Input: part model. Units: mm. Frame: model coordinates. A direction names the side the tool comes from. Coordinates: 2 decimals unless noted, no trailing zeros. Order: outer loops, then holes, each group sorted by start corner. A loop starts at its lowest first (then second) coordinate and runs counter-clockwise, first axis right, second up. Notation, with made-up numbers: (63, 83.5) -> (70, 83.5) arc R26 ccw to (70, 120.5) -> close; hole circle Ø4 at (79, 22.5). An arc over 180 degrees is marked (long way). Use one line per item in the form item = value. Start each with the question number.
1) Section query D-D on z = -7.5. Output: boundary loops of the cut face in (x, y), then the cut area to 3 significant figures.
2) Pin query (flat end, axial travel): pin 1 (5.5 mm diameter, centred on y = 9, z = -8, fed in from +X); pin 2 (7.5 mm diameter, centred on x = 5.5, y = 9.5, fed in from -Z); pin 3 (5 mm diameter, centred on x = -4, y = 8, fed in from -Z). Return the tip coordinate at first contact, or that it passes through.
3) Section query A-A on y = 14.25. Output: boundary loops of the cut face in (x, z), then the cut area to 3 significant figures.
4) Section query B-B on x = -21.5. Output: boundary loops of the cut face in (y, z), then the cut area to 3 significant figures.
5) Section query C-C on y = 3. Output: boundary loops of the cut face in (x, z).
6) Ray query, line 1 along X through (y, z) = (2.55, -18); line 2 along Y through (x, z) = (4, 4.5); line 3 along X through (y, z) = (12.5, 9). Return the intervals inside material, ascending.
7) Access query for faces 1 (the flat face through (-17, 10, 14)), 2 (the flat face through (-15, 10, 18.5)), 3 (the flat face through (15, 10, 16)), 4 (the flat face through (10, 10, 13.5)), 5 (the flat face through (17, 10, -1.5)). Directions: +Z, -Z, +X, -X, +Y, -Y. A direction counts if a zero-diameter tool reaches every point of the face in a straight line with its end or side. Return the directions, or none.
from build123d import *

# Parameters (mm, degrees)
ESQUISSE1_W        = 50
ESQUISSE1_H        = 43
ESQUISSE1_R        = 2
BOSS_EXTRU_1_DEPTH = 5
ESQUISSE2_W        = 5
ESQUISSE2_H        = 10
ESQUISSE2_H_2      = 7
ESQUISSE2_W_2      = 7
ESQUISSE2_H_3      = 5
ESQUISSE2_H_4      = 11
ESQUISSE2_W_3      = 10
BOSS_EXTRU_2_DEPTH = 15


with BuildPart() as part:
    # Esquisse1 → Boss.-Extru.1 (new body)
    with BuildSketch(Plane(origin=(0, 0, 0), x_dir=(1, 0, 0), z_dir=(0, 1, 0))):
        Rectangle(ESQUISSE1_W, ESQUISSE1_H)
        with Locations(Location((-21.5, 18, 0), (0, 0, 270))):
            Circle(ESQUISSE1_R, mode=Mode.SUBTRACT)
        with Locations(Location((21.5, 18, 0), (0, 0, 90))):
            Circle(ESQUISSE1_R, mode=Mode.SUBTRACT)
        with Locations(Location((21.5, -18, 0), (0, 0, 270))):
            Circle(ESQUISSE1_R, mode=Mode.SUBTRACT)
        with Locations(Location((-21.5, -18, 0), (0, 0, 90))):
            Circle(ESQUISSE1_R, mode=Mode.SUBTRACT)
    extrude(amount=BOSS_EXTRU_1_DEPTH)

    # Esquisse2 → Boss.-Extru.2 (add)
    with BuildSketch(Plane(origin=(0, 0, 0), x_dir=(1, 0, 0), z_dir=(0, 1, 0))):
        with Locations((-14.5, -13.5)):
            Rectangle(ESQUISSE2_W, ESQUISSE2_H)
        with Locations((-14.5, 8)):
            Rectangle(ESQUISSE2_W, ESQUISSE2_H_2)
        with Locations((4.5, 16)):
            Rectangle(ESQUISSE2_W_2, ESQUISSE2_H_3)
        with Locations((17.5, -4)):
            Rectangle(ESQUISSE2_W_2, ESQUISSE2_H_4)
        with Locations((10, -16)):
            Rectangle(ESQUISSE2_W_3, ESQUISSE2_H_3)
        with Locations((-3, -16)):
            Rectangle(ESQUISSE2_W_3, ESQUISSE2_H_3)
    extrude(amount=BOSS_EXTRU_2_DEPTH)


solid = part.part
Answers below:
q1.outline = (-25, 0) -> (25, 0) -> (25, 5) -> (-12, 5) -> (-12, 15) -> (-17, 15) -> (-17, 5) -> (-25, 5) -> close
q1.area = 300 mm^2
q2.pin_1 = -12
q2.pin_2 = -18.5
q2.pin_3 = 13.5
q3.outline = (-17, -11.5) -> (-12, -11.5) -> (-12, -4.5) -> (-17, -4.5) -> close; (-17, 8.5) -> (-12, 8.5) -> (-12, 18.5) -> (-17, 18.5) -> close; (-8, 13.5) -> (2, 13.5) -> (2, 18.5) -> (-8, 18.5) -> close; (1, -18.5) -> (8, -18.5) -> (8, -13.5) -> (1, -13.5) -> close; (5, 13.5) -> (15, 13.5) -> (15, 18.5) -> (5, 18.5) -> close; (14, -1.5) -> (21, -1.5) -> (21, 9.5) -> (14, 9.5) -> close
q3.area = 297 mm^2
q4.outline = (0, -21.5) -> (5, -21.5) -> (5, -20) -> (0, -20) -> close; (0, -16) -> (5, -16) -> (5, 16) -> (0, 16) -> close; (0, 20) -> (5, 20) -> (5, 21.5) -> (0, 21.5) -> close
q4.area = 175 mm^2
q5.outline = (-25, -21.5) -> (25, -21.5) -> (25, 21.5) -> (-25, 21.5) -> close; hole circle Ø4 at (-21.5, -18); hole circle Ø4 at (-21.5, 18); hole circle Ø4 at (21.5, -18); hole circle Ø4 at (21.5, 18)
q6.line_1 = -25 to -23.5, -19.5 to 19.5, 23.5 to 25
q6.line_2 = 0 to 5
q6.line_3 = -17 to -12, 14 to 21
q7.face_1 = +Z, -Z, -X, +Y
q7.face_2 = +Z, +X, -X, +Y
q7.face_3 = +Z, +X, +Y
q7.face_4 = +X, +Y
q7.face_5 = -Z, +X, -X, +Y
